Here's how the part is built. I have some questions about the finished solid (model axes, mm). A direction names the side the tool comes from. Coordinates: 2 decimals unless noted, no trailing zeros. Loops run counter-clockwise (first coordinate to the right, second up) from the corner with the lowest first, then second, coordinate; pieces in that order, holes last. Notation, with made-up numbers: (57.25, 50) -> (78.25, 50) arc R14 cw to (78.25, 68) -> close; hole circle Ø8 at (-3.75, 7). An arc over 180 degrees is marked (long way). Use CSV: the item, a comma, the result in double quotes. Start each with the question number.
from build123d import *

# Parameters (mm, degrees)
SKETCH1_R           = 8
BOSS_EXTRUDE1_DEPTH = 10.5
SKETCH2_R           = 3.85
BOSS_EXTRUDE2_DEPTH = 60
BOSS_EXTRUDE3_START = -9.6
BOSS_EXTRUDE3_DEPTH = 10
CUT_EXTRUDE1_START  = -9.6
SKETCH6_R           = 3.85
CUT_EXTRUDE1_DEPTH  = 9.6
BOSS_EXTRUDE4_DEPTH = 10
SKETCH8_R           = 4.5
BOSS_EXTRUDE5_DEPTH = 0.5
SKETCH9_R           = 3.85
BOSS_EXTRUDE6_DEPTH = 50.4
SKETCH11_W          = 7.6994
SKETCH11_H          = 9.7
BOSS_EXTRUDE7_DEPTH = 43.5
SKETCH12_R          = 1.75
CUT_EXTRUDE2_DEPTH  = 10


with BuildPart() as part:
    # Sketch1 → Boss-Extrude1 (new body)
    with BuildSketch(Plane.XY):
        Circle(SKETCH1_R)
    extrude(amount=-BOSS_EXTRUDE1_DEPTH)

    # Sketch2 → Boss-Extrude2 (add)
    with BuildSketch(Plane(origin=(0, 0, -10.5), x_dir=(-1, 0, 0), z_dir=(0, 0, -1))):
        Circle(SKETCH2_R)
    extrude(amount=BOSS_EXTRUDE2_DEPTH)

    # Sketch3 → Boss-Extrude3 (add)
    with BuildSketch(Plane(origin=(0, 0, -70.5), x_dir=(-1, 0, 0), z_dir=(0, 0, -1)).offset(BOSS_EXTRUDE3_START)):
        Polygon((-6, 1), (-1, 1), (-1, 6), (1, 6), (1, 1), (6, 1), (6, -1), (1, -1), (1, -6), (-1, -6), (-1, -1), (-6, -1), align=None)
    extrude(amount=-BOSS_EXTRUDE3_DEPTH)

    # Sketch6 → Cut-Extrude1 (cut)
    with BuildSketch(Plane(origin=(0, 0, -70.5), x_dir=(-1, 0, 0), z_dir=(0, 0, -1)).offset(CUT_EXTRUDE1_START)):
        with Locations(Location((0, 0, 0), (0, 0, 195.05465064))):
            Circle(SKETCH6_R)
    extrude(amount=CUT_EXTRUDE1_DEPTH, mode=Mode.SUBTRACT)

    # Sketch7 → Boss-Extrude4 (add)
    with BuildSketch(Plane.XY):
        with BuildLine():
            Line((-7.5, 72), (-7.5, 2.783882181))
            Line((-7.5, 2.783882181), (7.5, 2.783882181))
            Line((7.5, 2.783882181), (7.5, 72))
            ThreePointArc((7.5, 72), (0, 79.5), (-7.5, 72))
        make_face()
    extrude(amount=-BOSS_EXTRUDE4_DEPTH)

    # Sketch8 → Boss-Extrude5 (add)
    with BuildSketch(Plane(origin=(0, 0, -10), x_dir=(-1, 0, 0), z_dir=(0, 0, -1))):
        with Locations(Location((0, 72, 0), (0, 0, 180))):
            Circle(SKETCH8_R)
    extrude(amount=BOSS_EXTRUDE5_DEPTH)

    # Sketch9 → Boss-Extrude6 (add)
    with BuildSketch(Plane(origin=(0, 0, -10.5), x_dir=(-1, 0, 0), z_dir=(0, 0, -1))):
        with Locations(Location((0, 72, 0), (0, 0, 180))):
            Circle(SKETCH9_R)
    extrude(amount=BOSS_EXTRUDE6_DEPTH)

    # Sketch11 → Boss-Extrude7 (add)
    with BuildSketch(Plane(origin=(0, 0, -10), x_dir=(-1, 0, 0), z_dir=(0, 0, -1))):
        with Locations((-0.0003, 47)):
            Rectangle(SKETCH11_W, SKETCH11_H)
    extrude(amount=BOSS_EXTRUDE7_DEPTH)

    # Sketch12 → Cut-Extrude2 (cut)
    with BuildSketch(Plane(origin=(0, 0, -53.5), x_dir=(-1, 0, 0), z_dir=(0, 0, -1))):
        with Locations((-0.0003, 47)):
            Circle(SKETCH12_R)
    extrude(amount=-CUT_EXTRUDE2_DEPTH, mode=Mode.SUBTRACT)


solid = part.part
1) I want a section at B-B, the plane z = -32. Please give me the cut outline in (x, y).
2) Please list where these lines run through material, in increasing order: L1, parallel to Y at x = -1.75, z = -11.5; L2, parallel to Y at x = 1, z = -33; L3, parallel to Z at x = 2, y = 37. Write a range as [from, to].
3) I want a section at C-C, the plane y = 0. Please give me the cut outline in (x, z).
4) I want a section at D-D, the plane z = -8. Please give me the cut outline in (x, y), plus the area to 3 significant figures.
5) Thinking about a two-plate mould opening in Y: for faces 1 (the face through (7.5, 37, -5)), 2 (the face through (-0.83, 75.76, -35.35)), 3 (the face through (0, 6, -56)), 4 (the face through (-5, -1, -56)), which applies, pulls with the +Y half, pulls with the -Y half, needs draft (parallel to the pull), parting line crosses it, or undercut?
6) Which directions (+Z, -Z, +X, -X, +Y, -Y) give clear straight access to the entire face, cutting with the end or side of a thin tool? Please do faces 5 (the face through (0.38, 45.29, -48.57)), 6 (the face through (5, -1, -56)), 7 (the face through (0, 51.85, -31)), 8 (the face through (-6, 0, -56)).
7) I want a section at A-A, the plane z = -45.5. Please give me the cut outline in (x, y), plus the area to 3 significant figures.
8) For P1, Ø8, axis at x = 0.5, z = -43.5, coming from the -Y side; P2, Ø2, axis at x = 0, z = -54.5, coming from the -Y side; P3, Ø1, axis at x = -0.5, y = -4.5, coming from the +Z side; P4, Ø1.1, axis at x = -5, z = -55.5, coming from the -Y side, each with a flat end and sliding along its axis, tell me the tip position at first contact or that it passes through.
Return value:
1,outline,"circle Ø7.7 at (0, 0); (-3.85, 42.15) -> (3.85, 42.15) -> (3.85, 51.85) -> (-3.85, 51.85) -> close; circle Ø7.7 at (0, 72)"
2,L1,"y = [-3.43, 3.43], [42.15, 51.85], [68.57, 75.43]"
2,L2,"y = [-3.72, 3.72], [42.15, 51.85], [68.28, 75.72]"
2,L3,"z = [-10, 0]"
3,outline,"(-8, -10.5) -> (-3.85, -10.5) -> (-3.85, -50.9) -> (-6, -50.9) -> (-6, -60.9) -> (6, -60.9) -> (6, -50.9) -> (3.85, -50.9) -> (3.85, -10.5) -> (8, -10.5) -> (8, 0) -> (-8, 0) -> close"
4,outline,"(-7.5, 2.78) arc R8 ccw (long way) to (7.5, 2.78) -> (7.5, 72) arc R7.5 ccw to (-7.5, 72) -> close"
4,area,"1,270 mm²"
5,face 1,"needs draft"
5,face 2,"undercut"
5,face 3,"undercut"
5,face 4,"pulls with the -Y half"
6,face 5,"-Z"
6,face 6,"-Z, +X, -Y"
6,face 7,"-Z, +X, -X"
6,face 8,"-Z, -X, +Y, -Y"
7,outline,"circle Ø7.7 at (0, 0); (-3.85, 42.15) -> (3.85, 42.15) -> (3.85, 51.85) -> (-3.85, 51.85) -> close; circle Ø7.7 at (0, 72); hole circle Ø3.5 at (0, 47)"
7,area,"158 mm²"
8,P1,"stops at y = -3.85"
8,P2,"stops at y = -6"
8,P3,"stops at z = 0"
8,P4,"stops at y = -1"
